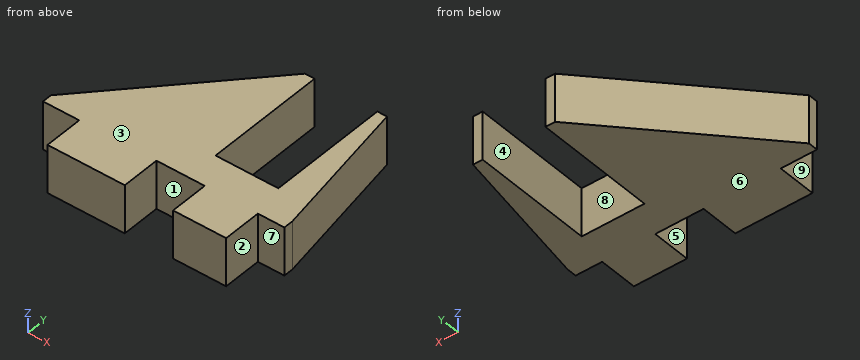
Autodesk Inventor part; units mm, degrees
ref_plane "YZ Plane" through (0, 0, 0) normal (1, 0, 0) x (0, 1, 0)
ref_plane "XZ Plane" through (0, 0, 0) normal (0, 1, 0) x (-1, 0, 0)
ref_plane "XY Plane" through (0, 0, 0) normal (0, 0, 1) x (1, 0, 0)
sketch "Esquisse1" plane through (0, 0, 0) normal (0, 0, 1) x (1, 0, 0)
  line L0 (50, 0) -> (50, 2)
  line L1 (0, 2) -> (0, 0)
  line L2 (43, 32) -> (43, 7)
  line L3 (43, 7) -> (30, 7)
  line L4 (30, 7) -> (30, 32)
  line L5 (28, 32) -> (30, 32)
  line L6 (43, 32) -> (45, 32)
  line L7 (0, 2) -> (50, 2) construction
  line L8 (0, 2) -> (28, 32)
  line L9 (45, 32) -> (50, 2)
  line L10 (23.5, 0) -> (23.5, -8)
  line L11 (23.5, -8) -> (7.5, -8)
  line L12 (7.5, -8) -> (7.5, 0)
  line L13 (44.5, 0) -> (44.5, -8)
  line L14 (44.5, -8) -> (33.5, -8)
  line L15 (33.5, -8) -> (33.5, 0)
  line L16 (0, 0) -> (7.5, 0)
  line L17 (23.5, 0) -> (33.5, 0)
  line L18 (44.5, 0) -> (50, 0)
  dimension "d10" = 50
  dimension "d12" = 13
  dimension "d13" = 7
  dimension "d14" = 25
  dimension "d15" = 25
  dimension "d21" = 16
  dimension "d23" = 7.5
  dimension "d24" = 11
  dimension "d26" = 5.5
  dimension "d27" = 7
  dimension "d28" = 8
  dimension "d29" = 8
  dimension "d30" = 8
  dimension "d31" = 8
  dimension "d34" = 80.538
  dimension "d35" = 30
  dimension "d36" = 46.975
extrude "Extrusion1" add sketch "Esquisse1" along normal blind 10
properties part number "Support_motor_front_ground"
Work out the finished part from the listing and answer in its coordinate system (mm). Face numbers are marked on the shaded views. A direction names the side the tool comes from. Give positions to 0.01 mm unless a question says otherwise; leave off trailing zeros. Write each loop counter-clockwise with the first axis right and the second up, starting at its lowest first coordinate (ties: lowest second). Pieces come first, ordered by that corner, then holes.
(1) Straight lines are drawn through the part: line 1 (X direction, y = -1.5, z = 2); line 2 (X direction, y = 29, z = 4.5); line 3 (Y direction, x = 40.5, z = 1.5). For each, find the intervals that lie inside material, in ascending order.
Final values:
line 1: x = 7.5 to 23.5, 33.5 to 44.5
line 2: x = 25.2 to 30, 43 to 45.5
line 3: y = -8 to 7
(2) Flat-ended cylindrical pins translate along their axes: pin 1 Ø5 at (y, z) = (6, 3.5) entering from +X; pin 2 Ø1.6 at (x, z) = (46, 3.5) entering from -Y; pin 3 Ø5 at (y, z) = (19.5, 5) entering from -X. Find the tip coordinate at first contact, or state that the pin passes through.
Final values:
pin 1: stops at x = 49.75
pin 2: stops at y = 0
pin 3: stops at x = 14
(3) Which of the six approach directions +Z, -Z, +X, -X, +Y, -Y give full straight-line access (tool end or side, diameter ignored) to the marked faces 5, 6, 7, 8 and 9?
Final values:
face 5: +Z, -Z, -Y
face 6: -Z, +X, -X, +Y, -Y
face 7: +Z, -Z, +X, -Y
face 8: +Z, -Z, +Y
face 9: +Z, -Z, -X, -Y
(4) The mould has two halves that part along X. Classify the marked faces 1, 2, 3 and 4: pulls with the +X half, pulls with the -X half, needs draft (parallel to the pull), parting line crosses it, or undercut.
Final values:
face 1: undercut
face 2: pulls with the +X half
face 3: needs draft
face 4: undercut
(5) The part is cut by section A-A on y = 25.5. Write down the section's boundary in (x, z), plus the area to 4 significant figures.
Final values:
outline: (21.93, 0) - (30, 0) - (30, 10) - (21.93, 10) - close; (43, 0) - (46.08, 0) - (46.08, 10) - (43, 10) - close
area: 111.5 mm2
(6) The part is cut by section C-C on y = 21. Write down the section's boundary in (x, z), plus the area to 3 significant figures.
Final values:
outline: (17.73, 0) - (30, 0) - (30, 10) - (17.73, 10) - close; (43, 0) - (46.83, 0) - (46.83, 10) - (43, 10) - close
area: 161 mm2
(7) The part is cut by section D-D on x = 31.5. Write down the section's boundary in (y, z), plus the area to 3 significant figures.
Final values:
outline: (0, 0) - (7, 0) - (7, 10) - (0, 10) - close
area: 70.0 mm2
(8) The part is cut by section B-B on z = 5. Write down the section's boundary in (x, y).
Final values:
outline: (0, 0) - (7.5, 0) - (7.5, -8) - (23.5, -8) - (23.5, 0) - (33.5, 0) - (33.5, -8) - (44.5, -8) - (44.5, 0) - (50, 0) - (50, 2) - (45, 32) - (43, 32) - (43, 7) - (30, 7) - (30, 32) - (28, 32) - (0, 2) - close
